Build history of the part. All positions in model axes, mm. Face numbers are marked on the shaded views. A direction names the side the tool comes from. Give positions to 0.01 mm unless a question says otherwise; leave off trailing zeros. Write each loop counter-clockwise with the first axis right and the second up, starting at its lowest first coordinate (ties: lowest second). Pieces come first, ordered by that corner, then holes. Notation, with made-up numbers: (-14, 15.25) -> (-3, 15.25) arc R12 cw to (-3, 28.25) -> close; hole circle Ø3 at (0, 52). An arc over 180 degrees is marked (long way). Put each result on its own line as item: value.
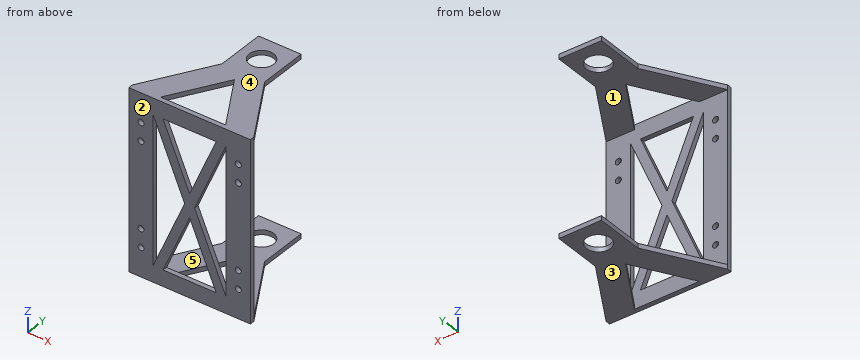
Autodesk Inventor part; units mm, degrees
ref_plane "Work Plane2" through (0, 0, 177.8) normal (0, 0, 1) x (1, 0, 0)
ref_plane "YZ Plane" through (0, 0, 0) normal (1, 0, 0) x (0, 1, 0)
ref_plane "XZ Plane" through (0, 0, 0) normal (0, 1, 0) x (-1, 0, 0)
sketch "Sketch1" plane through (0, 0, 0) normal (0, 1, 0) x (-1, 0, 0)
  line L0 (-127, 228.6) -> (-127, -228.6)
  line L1 (-65.8371, -177.8) -> (65.8371, -177.8)
  line L2 (127, -228.6) -> (127, 228.6)
  line L3 (65.8371, 177.8) -> (-65.8371, 177.8)
  line L4 (127, -228.6) -> (-127, -228.6)
  line L5 (-127, 228.6) -> (127, 228.6)
  line L6 (-76.2, 153.6199) -> (-76.2, -153.6199)
  line L7 (76.2, -153.6199) -> (76.2, 153.6199)
  line L8 (76.2, -153.6199) -> (10.3629, 0)
  line L9 (0, 24.1801) -> (-65.8371, 177.8)
  line L10 (65.8371, -177.8) -> (0, -24.1801)
  line L11 (-10.3629, 0) -> (-76.2, 153.6199)
  line L12 (76.2, 153.6199) -> (10.3629, 0)
  line L13 (0, -24.1801) -> (-65.8371, -177.8)
  line L14 (65.8371, 177.8) -> (0, 24.1801)
  line L15 (-10.3629, 0) -> (-76.2, -153.6199)
  point P0 (0, 0)
  point P1 (-127, 155.9501)
  point P2 (127, -155.9501)
  point P3 (-127, -155.9501)
  point P4 (127, 155.9501)
extrude "Extrusion3" add sketch "Sketch1" along normal blind 9.525
sketch "Sketch7" plane through (0, 9.525, 0) normal (0, 1, 0) x (1, 0, 0)
  line L0 (0, 24.1801) -> (-65.8371, 177.8)
  line L1 (-127, 228.6) -> (-127, -228.6)
  line L2 (-76.2, 153.6199) -> (-76.2, -153.6199)
  circle A0 centre (-101.6, 127) radius 6.35
  circle A1 centre (-101.6, 88.9) radius 6.35
  line L3 (127, 228.6) -> (-127, 228.6)
  line L4 (-127, -228.6) -> (127, -228.6)
  circle A2 centre (101.6, 127) radius 6.35
  circle A3 centre (101.6, 88.9) radius 6.35
  line L5 (127, -228.6) -> (127, 228.6)
  circle A4 centre (-101.6, -127) radius 6.35
  circle A5 centre (-101.6, -88.9) radius 6.35
  circle A6 centre (101.6, -127) radius 6.35
  circle A7 centre (101.6, -88.9) radius 6.35
  point P0 (0, 0)
extrude "Extrusion4" cut sketch "Sketch7" against normal up to next contours A0 | A1 | A2 | A3 | A4 | A5 | A6 | A7
sketch "Sketch8" plane through (127, 0, -228.6) normal (0, 0, -1) x (-1, 0, 0)
  point P0 (127, 0)
ref_plane "Work Plane2" through (0, 0, 177.8) normal (0, 0, 1) x (1, 0, 0)
mirror "Mirror3" about plane through (0, 0, 0) normal (0, 0, 1)
sketch "Sketch13" plane through (0, 0, 177.8) normal (0, 0, 1) x (1, 0, 0)
  line L0 (0, 0) -> (0, 9.525)
  line L1 (-127, 9.525) -> (127, 9.525)
  line L2 (0, 9.525) -> (-44.45, 9.525)
  line L3 (-44.45, 250.825) -> (44.45, 250.825)
  circle A0 centre (0, 200.025) radius 25.4
  line L4 (-127, 0) -> (-127, 9.525)
  line L5 (-44.45, 149.225) -> (-127, 9.525)
  line L6 (127, 0) -> (127, 9.525)
  line L7 (44.45, 149.225) -> (127, 9.525)
  line L8 (67.9938, 9.525) -> (0, 124.5914)
  line L9 (0, 124.5914) -> (-67.9938, 9.525)
  line L10 (44.45, 250.825) -> (44.45, 149.225)
  line L11 (-44.45, 149.225) -> (-44.45, 250.825)
  dimension "d52" = 88.9
  dimension "d56" = 50.8
  dimension "d57" = 50.8
extrude "Extrusion8" add sketch "Sketch13" along normal blind 9.525 contours L5 L11 L3 L10 L7 L1 L8 L9
mirror "Mirror4" about plane through (0, 0, 0) normal (0, 0, 1) of "Extrusion8"
sketch "Sketch14" plane through (0, 9.525, 0) normal (0, 1, 0) x (1, 0, 0)
  line L0 (-127, 228.6) -> (-127, 187.325)
  line L1 (67.9938, 187.325) -> (127, 187.325)
  line L2 (-127, 228.6) -> (127, 228.6)
  line L3 (127, 228.6) -> (127, 187.325)
  line L4 (127, 187.325) -> (-127, 187.325)
  line L5 (-127, 187.325) -> (-127, 228.6)
  line L6 (-44.45, -187.325) -> (-127, -187.325)
  line L7 (-127, -228.6) -> (127, -228.6)
  line L8 (-127, -187.325) -> (127, -187.325)
  line L9 (127, -187.325) -> (127, -228.6)
  line L10 (127, -228.6) -> (-127, -228.6)
  line L11 (-127, -228.6) -> (-127, -187.325)
  point P0 (0, 0)
extrude "Extrusion9" cut sketch "Sketch14" against normal blind 25.4
sketch "Sketch15" plane through (0, 9.525, 0) normal (0, 1, 0) x (1, 0, 0)
  line L0 (-76.2, 153.6199) -> (-10.3629, 0)
  line L1 (-76.2, 153.6199) -> (76.2, 153.6199)
  line L2 (76.2, 153.6199) -> (76.2, 177.8)
  line L3 (127, 177.8) -> (44.45, 177.8)
  line L4 (-76.2, 153.6199) -> (-76.2, 177.8)
  line L5 (-76.2, 177.8) -> (76.2, 177.8)
  line L6 (-44.45, -177.8) -> (-127, -177.8)
  line L7 (-76.2, -177.8) -> (76.2, -177.8)
  line L8 (76.2, -177.8) -> (76.2, -152.9852)
  line L9 (76.2, -152.9852) -> (-76.2, -152.9852)
  line L10 (-76.2, -152.9852) -> (-76.2, -177.8)
  point P0 (0, 0)
extrude "Extrusion10" add sketch "Sketch15" against normal blind 9.525 contours L4 L5 L3 L2 L1
sketch "Sketch16" plane through (0, 9.525, 0) normal (0, 1, 0) x (1, 0, 0)
  line L0 (-76.2, -153.6199) -> (-10.3629, 0)
  line L1 (-76.2, -153.6199) -> (-76.2, -177.8)
  line L2 (-127, -177.8) -> (-67.9938, -177.8)
  line L3 (76.2, -153.6199) -> (76.2, 153.6199)
  line L4 (76.2, -153.6199) -> (-76.2, -153.6199)
  line L5 (-76.2, -153.6199) -> (-76.2, -177.8)
  line L6 (-76.2, -177.8) -> (76.2, -177.8)
  line L7 (76.2, -177.8) -> (76.2, -153.6199)
  point P0 (0, 0)
extrude "Extrusion11" add sketch "Sketch16" against normal blind 9.525
ref_plane "Work Plane3" through (0, 0, 0) normal (0, 0, 1) x (1, 0, 0)
properties part number "Square Support"
1) Pull direction Z, two halves, no side cores. Call the marked faces 1, 2 and 3: released by +Z, released by -Z, zero draft, split by the parting line, or undercut.
Filled sheet:
face 1: undercut
face 2: zero draft
face 3: released by -Z
2) Slice it at C-C (y = 56). Write the cut outline in (x, z) (1 decimal).
Filled sheet:
outline: (-99.5, -187.3) -> (-40.5, -187.3) -> (-40.5, -177.8) -> (-99.5, -177.8) -> close; (-99.5, 177.8) -> (-40.5, 177.8) -> (-40.5, 187.3) -> (-99.5, 187.3) -> close; (40.5, -187.3) -> (99.5, -187.3) -> (99.5, -177.8) -> (40.5, -177.8) -> close; (40.5, 177.8) -> (99.5, 177.8) -> (99.5, 187.3) -> (40.5, 187.3) -> close
3) Wall check: L1, parallel to Z at x = -101.6, y = 4.5 (3 decimals); L2, parallel to Z at x = 44.5, y = 126 (3 decimals); L3, parallel to Y at x = -83.5, z = -153 (3 decimals). Give the ranges that are in metal, low to high.
Filled sheet:
L1: -187.325 to -133.35, -120.65 to -95.25, -82.55 to 82.55, 95.25 to 120.65, 133.35 to 187.325
L2: -187.325 to -177.8, 177.8 to 187.325
L3: 0 to 9.525
4) Tool access for the marked faces 4 and 5: list every direction of +Z, -Z, +X, -X, +Y, -Y with a clear straight run to the whole face (end or side of a thin tool).
Filled sheet:
face 4: +Z, +X, -X, +Y, -Y
face 5: +X, -X, +Y
5) Slice it at D-D (z = 88.9). Write the cut outline in (x, y) (3 decimals), plus the area to 3 significant figures.
Filled sheet:
outline: (-127, 0) -> (-107.95, 0) -> (-107.95, 9.525) -> (-127, 9.525) -> close; (-95.25, 0) -> (-76.2, 0) -> (-76.2, 9.525) -> (-95.25, 9.525) -> close; (-48.463, 0) -> (-27.737, 0) -> (-27.737, 9.525) -> (-48.463, 9.525) -> close; (27.737, 0) -> (48.463, 0) -> (48.463, 9.525) -> (27.737, 9.525) -> close; (76.2, 0) -> (95.25, 0) -> (95.25, 9.525) -> (76.2, 9.525) -> close; (107.95, 0) -> (127, 0) -> (127, 9.525) -> (107.95, 9.525) -> close
area: 1,120 mm2
6) Slice it at B-B (x = -49). Write the cut outline in (y, z) (3 decimals).
Filled sheet:
outline: (0, -187.325) -> (9.525, -187.325) -> (9.525, -153.62) -> (0, -153.62) -> close; (0, -138.513) -> (9.525, -138.513) -> (9.525, -90.153) -> (0, -90.153) -> close; (0, 90.153) -> (9.525, 90.153) -> (9.525, 138.513) -> (0, 138.513) -> close; (0, 153.62) -> (9.525, 153.62) -> (9.525, 187.325) -> (0, 187.325) -> close; (41.668, -187.325) -> (141.525, -187.325) -> (141.525, -177.8) -> (41.668, -177.8) -> close; (41.668, 177.8) -> (141.525, 177.8) -> (141.525, 187.325) -> (41.668, 187.325) -> close
7) Pin check, flat tips, straight feed: pin 1 (7.5 mm diameter, centred on y = 207, z = -182.5, fed in from +X); pin 2 (6 mm diameter, centred on x = -87.5, z = -38.5, fed in from +Y) (3 decimals); pin 3 (3 mm diameter, centred on y = 176.5, z = -181, fed in from -X). Stop position of each tip, or through.
Filled sheet:
pin 1: x = 44.45
pin 2: y = 9.525
pin 3: x = -44.45
8) Slice it at A-A (y = 138). Write the cut outline in (x, z) (3 decimals), plus the area to 3 significant figures.
Filled sheet:
outline: (-51.083, -187.325) -> (51.083, -187.325) -> (51.083, -177.8) -> (-51.083, -177.8) -> close; (-51.083, 177.8) -> (51.083, 177.8) -> (51.083, 187.325) -> (-51.083, 187.325) -> close
area: 1,950 mm2
